from build123d import *

# Parameters (mm, degrees)
EXTRUDE_1_DEPTH     = 50
SKETCH_2_R          = 2.5
EXTRUDE_2_DEPTH     = 5
CUT_EXTRUDE_2_DEPTH = 2
SKETCH_7_W          = 132
SKETCH_7_H          = 55
EXTRUDE_3_DEPTH     = 5
SKETCH_8_W          = 122
SKETCH_8_H          = 5
CUT_EXTRUDE_3_DEPTH = 50
EXTRUDE_4_DEPTH     = 5
FILLET_1_R          = 10
FILLET_2_R          = 10
FILLET_3_R          = 10
FILLET_4_R          = 10
FILLET_5_R          = 10
FILLET_6_R          = 10
FILLET_7_R          = 10
FILLET_8_R          = 10


with BuildPart() as part:
    # 草图1 → 凸台-拉伸1 (new body)
    with BuildSketch(Plane.XY):
        Polygon((-66, 30), (66, 30), (66, -25), (61, -25), (61, 25), (-61, 25), (-61, -25), (-66, -25), align=None)
    extrude(amount=EXTRUDE_1_DEPTH)

    # 草图2 → 凸台-拉伸2 (add)
    # profile 1 of 2: a face of its own
    with BuildSketch(Plane.XY):
        with BuildLine():
            Line((-61, -13), (-53.5, -13))
            ThreePointArc((-53.5, -13), (-47.5, -19), (-53.5, -25))
            Line((-53.5, -25), (-61, -25))
            Line((-61, -25), (-61, -13))
        make_face()
        with Locations((-53.5, -19)):
            Circle(SKETCH_2_R, mode=Mode.SUBTRACT)
    # profile 2 of 2: a face of its own
    with BuildSketch(Plane.XY):
        with BuildLine():
            Line((61, -25), (53.5, -25))
            ThreePointArc((53.5, -25), (47.5, -19), (53.5, -13))
            Line((53.5, -13), (61, -13))
            Line((61, -13), (61, -25))
        make_face()
        with Locations((53.5, -19)):
            Circle(SKETCH_2_R, mode=Mode.SUBTRACT)
    extrude(amount=EXTRUDE_2_DEPTH)

    # 草图6 → 切除-拉伸2 (cut)
    with BuildSketch(Plane.XY.offset(5)):
        Polygon((-49.74722325, -19), (-51.623611625, -15.75), (-55.376388375, -15.75), (-57.25277675, -19), (-55.376388375, -22.25), (-51.623611625, -22.25), align=None)
        Polygon((57.25277675, -19), (55.376388375, -15.75), (51.623611625, -15.75), (49.74722325, -19), (51.623611625, -22.25), (55.376388375, -22.25), align=None)
    extrude(amount=-CUT_EXTRUDE_2_DEPTH, mode=Mode.SUBTRACT)

    # 草图7 → 凸台-拉伸3 (add)
    with BuildSketch(Plane.XY.offset(50)):
        with Locations((0, 2.5)):
            Rectangle(SKETCH_7_W, SKETCH_7_H)
    extrude(amount=EXTRUDE_3_DEPTH)

    # 草图8 → 切除-拉伸3 (cut)
    with BuildSketch(Plane(origin=(0, 0, 0), x_dir=(-1, 0, 0), z_dir=(0, 0, -1))):
        with Locations((0, 27.5)):
            Rectangle(SKETCH_8_W, SKETCH_8_H)
    extrude(amount=-CUT_EXTRUDE_3_DEPTH, mode=Mode.SUBTRACT)

    # 草图9 → 凸台-拉伸4 (add)
    with BuildSketch(Plane.XY.offset(55)):
        Polygon((-66, 30), (66, 30), (66, 70), (55, 95), (31, 95), (20, 70), (-20, 70), (-31, 95), (-55, 95), (-66, 70), align=None)
    extrude(amount=-EXTRUDE_4_DEPTH)

    # 圆角1
    fillet_1_edges = [part.edges().sort_by_distance(p)[0] for p in [
        (-66, 70, 52.5),
    ]]
    fillet(fillet_1_edges, radius=FILLET_1_R)

    # 圆角2
    fillet_2_edges = [part.edges().sort_by_distance(p)[0] for p in [
        (-55, 95, 52.5),
    ]]
    fillet(fillet_2_edges, radius=FILLET_2_R)

    # 圆角3
    fillet_3_edges = [part.edges().sort_by_distance(p)[0] for p in [
        (66, 70, 52.5),
    ]]
    fillet(fillet_3_edges, radius=FILLET_3_R)

    # 圆角4
    fillet_4_edges = [part.edges().sort_by_distance(p)[0] for p in [
        (-31, 95, 52.5),
    ]]
    fillet(fillet_4_edges, radius=FILLET_4_R)

    # 圆角5
    fillet_5_edges = [part.edges().sort_by_distance(p)[0] for p in [
        (-20, 70, 52.5),
    ]]
    fillet(fillet_5_edges, radius=FILLET_5_R)

    # 圆角6
    fillet_6_edges = [part.edges().sort_by_distance(p)[0] for p in [
        (20, 70, 52.5),
    ]]
    fillet(fillet_6_edges, radius=FILLET_6_R)

    # 圆角7
    fillet_7_edges = [part.edges().sort_by_distance(p)[0] for p in [
        (31, 95, 52.5),
    ]]
    fillet(fillet_7_edges, radius=FILLET_7_R)

    # 圆角8
    fillet_8_edges = [part.edges().sort_by_distance(p)[0] for p in [
        (55, 95, 52.5),
    ]]
    fillet(fillet_8_edges, radius=FILLET_8_R)


solid = part.part
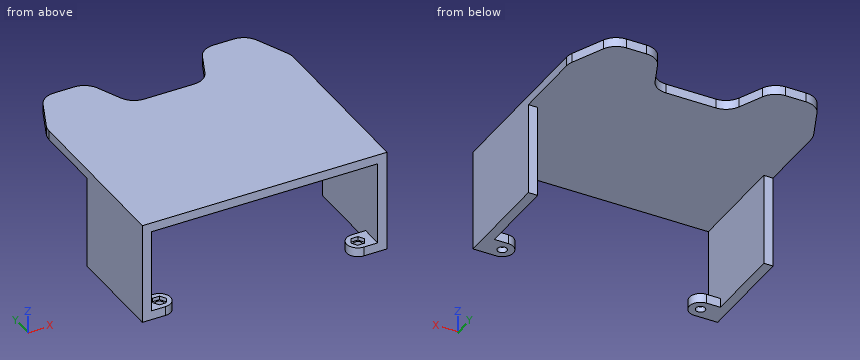
Could you check a few things on this model? Use its own coordinates, in mm. Coordinates: 2 decimals unless noted, no trailing zeros. Loops run counter-clockwise (first coordinate to the right, second up) from the corner with the lowest first, then second, coordinate; pieces in that order, holes last.
1. Imagine slicing it at B-B (y = 87). Please give me the cut outline in (x, z), and give its area (3 significant figures).
2. Imagine slicing it at C-C (y = 16). Please give me the cut outline in (x, z).
3. Imagine slicing it at D-D (x = 35). Please give me the cut outline in (y, z).
4. For P1, Ø4, axis at x = -64, z = 37, coming from the +Y side; P2, Ø1.5, axis at x = -58, z = 2.5, coming from the +Y side; P3, Ø5, axis at x = -9.5, y = -10.5, coming from the -Z side, each with a flat end and sliding along its axis, tell me the tip position at first contact or that it passes through.
5. Imagine slicing it at A-A (z = 22). Please give me the cut outline in (x, y), and give its area (3 significant figures).
6. I need wall thicknesses on L1, parallel to X at y = -19, z = 1.9; L2, parallel to X at y = -7.5, z = 43; L3, parallel to Y at x = -53.5, z = 1.8. Which ranges of each line are inside material? Lowest first, please.
Computed values:
1. outline: (-58.52, 50) - (-27.48, 50) - (-27.48, 55) - (-58.52, 55) - close; (27.48, 50) - (58.52, 50) - (58.52, 55) - (27.48, 55) - close
1. area: 310 mm2
2. outline: (-66, 0) - (-61, 0) - (-61, 50) - (61, 50) - (61, 0) - (66, 0) - (66, 55) - (-66, 55) - close
3. outline: (-25, 50) - (94.68, 50) - (94.68, 55) - (-25, 55) - close
4. P1: stops at y = 30
4. P2: stops at y = -13
4. P3: stops at z = 50
5. outline: (-66, -25) - (-61, -25) - (-61, 30) - (-66, 30) - close; (61, -25) - (66, -25) - (66, 30) - (61, 30) - close
5. area: 550 mm2
6. L1: x = -66 to -56, -51 to -47.5, 47.5 to 51, 56 to 66
6. L2: x = -66 to -61, 61 to 66
6. L3: y = -25 to -21.5, -16.5 to -13
